```python
from build123d import *

# Parameters (mm, degrees)
F1_DEPTH = 31.75
F2_R     = 15.875
F3_DEPTH = 80.823305
F4_R     = 12.7
F5_DEPTH = 63.501


with BuildPart() as f1:
    # F0 (on Front) → F1 (new body, symmetric)
    with BuildSketch(Plane.XZ):
        Polygon((0, 76.2), (0, 0), (76.2, 0), (76.2, 38.1), (38.1, 76.2), align=None)
    extrude(amount=F1_DEPTH, both=True)

    # F2 (on face) → F3 (cut, through all)
    with BuildSketch(Plane(origin=(57.15, 0, 57.15), x_dir=(0.707107, 0, -0.707107), z_dir=(0.707107, 0, 0.707107))):
        Circle(F2_R)
    extrude(amount=-F3_DEPTH, mode=Mode.SUBTRACT)

    # F4 (on face) → F5 (cut, through all)
    with BuildSketch(Plane.XZ.offset(31.75)):
        with Locations((30.563999, 36.636498)):
            Circle(F4_R)
    extrude(amount=-F5_DEPTH, mode=Mode.SUBTRACT)


solid = f1.part
```
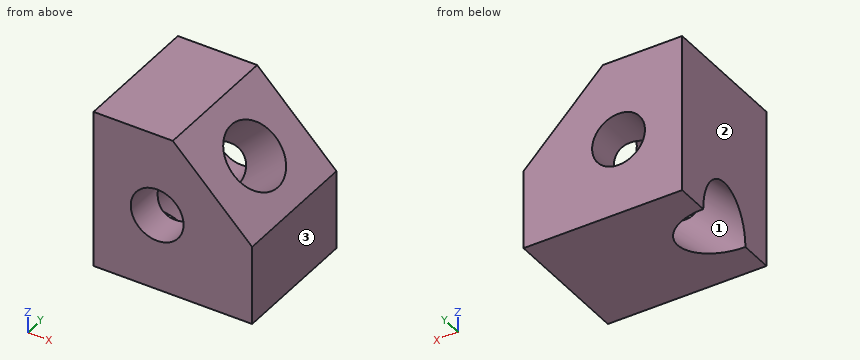
Could you check a few things on this model? Use its own coordinates, in mm. Face numbers are marked on the shaded views. Give positions to 0.01 mm unless a question says otherwise; leave off trailing zeros. Write each loop counter-clockwise with the first axis right and the second up, starting at its lowest first coordinate (ties: lowest second). Pieces come first, ordered by that corner, then holes. Notation, with made-up numbers: (-8, 24) - (3, 24) arc R5 ccw to (3, 30) - close; hole circle Ø7 at (43, 36.5). An arc over 180 degrees is marked (long way). One line per item, written item: value. Start each with the question number.
Item 1: Imagine slicing it at C-C, the plane y = 2.5. List the corners of the cut face in (x, z) for me, and give its area (3 significant figures).
Item 2: If we mould it in two halves opening along X, with no side actions, what happens to the marked faces 1, 2 and 3? For each: +X half, -X half, draft (parallel to the pull), parting line (faces both ways), or undercut.
Item 3: Imagine slicing it at A-A, the plane y = -13.5. List the corners of the cut face in (x, z) for me, and give its area (3 significant figures).
Item 4: Please list where these lines run through material, in increasing order: line 1 (X direction, y = -21, z = 37); line 2 (Y direction, x = 48.5, z = 35.5); line 3 (X direction, y = 11, z = 45). Write a range as from..to.
Item 5: Imagine slicing it at B-B, the plane y = 19.5. List the corners of the cut face in (x, z) for me.
Geometry says:
1. outline: (0, 22.17) - (18.53, 40.7) arc R12.7 cw to (26.5, 48.67) - (46.06, 68.24) - (38.1, 76.2) - (0, 76.2) - close; (22.17, 0) - (76.2, 0) - (76.2, 38.1) - (68.24, 46.06) - close
1. area: 2,780 mm^2
2. face 1: undercut
2. face 2: -X half
2. face 3: +X half
3. outline: (0, 11.81) - (19.18, 31) arc R12.7 cw to (36.2, 48.02) - (51.24, 63.06) - (38.1, 76.2) - (0, 76.2) - close; (11.81, 0) - (76.2, 0) - (76.2, 38.1) - (63.06, 51.24) - (40.33, 28.52) arc R12.7 cw to (38.68, 26.87) - close
3. area: 3,650 mm^2
4. line 1: 0..17.87, 43.26..76.2
4. line 2: -31.75..-12.94, 12.94..31.75
4. line 3: 0..21.01, 61.19..69.3
5. outline: (0, 0) - (76.2, 0) - (76.2, 38.1) - (38.1, 76.2) - (0, 76.2) - close; hole circle Ø25.4 at (30.56, 36.64)
